Could you check a few things on this model? Use its own coordinates, in mm. A direction names the side the tool comes from. Round coordinates to 2 decimals unless told otherwise and drop trailing zeros. Loops run counter-clockwise (first coordinate to the right, second up) from the corner with the lowest first, then second, coordinate; pieces in that order, holes last.
from build123d import *

# Parameters (mm, degrees)
SKETCH1_W               = 35.2
SKETCH1_H               = 35.2
BOSS_EXTRUDE1_DEPTH     = 34.8
SKETCH2_R               = 11.5
BOSS_EXTRUDE2_DEPTH     = 2
SKETCH3_R               = 2.5
BOSS_EXTRUDE3_DEPTH     = 23
SKETCH4_R               = 1.5
CUT_EXTRUDE1_DEPTH      = 8
MIRROR2_COPY_1_SKETCH_R = 1.5
MIRROR2_COPY_1_DEPTH    = 8
CUT_EXTRUDE2_DEPTH      = 6.96
MIRROR4_COPY_1_DEPTH    = 6.96
CUT_EXTRUDE3_DEPTH      = 6.96
MIRROR6_COPY_1_DEPTH    = 6.96
SKETCH7_R               = 2.5
CUT_EXTRUDE4_DEPTH      = 5
CUT_EXTRUDE6_DEPTH      = 20.88
CUT_EXTRUDE7_DEPTH      = 20.88
CUT_EXTRUDE8_DEPTH      = 20.88
CUT_EXTRUDE9_DEPTH      = 20.88


with BuildPart() as part:
    # Sketch1 → Boss-Extrude1 (new body)
    with BuildSketch(Plane(origin=(0, 0, 0), x_dir=(1, 0, 0), z_dir=(0, 1, 0))):
        Rectangle(SKETCH1_W, SKETCH1_H)
    extrude(amount=BOSS_EXTRUDE1_DEPTH)

    # Sketch2 → Boss-Extrude2 (add)
    with BuildSketch(Plane(origin=(0, 34.8, 0), x_dir=(1, 0, 0), z_dir=(0, 1, 0))):
        Circle(SKETCH2_R)
    extrude(amount=BOSS_EXTRUDE2_DEPTH)

    # Sketch3 → Boss-Extrude3 (add)
    with BuildSketch(Plane(origin=(0, 36.8, 0), x_dir=(1, 0, 0), z_dir=(0, 1, 0))):
        Circle(SKETCH3_R)
    extrude(amount=BOSS_EXTRUDE3_DEPTH)

    # Sketch4 → Cut-Extrude1 (cut)
    with BuildSketch(Plane(origin=(0, 34.8, 0), x_dir=(1, 0, 0), z_dir=(0, 1, 0))):
        with Locations((-13.1, 13.1)):
            Circle(SKETCH4_R)
    cut_extrude1 = extrude(amount=-CUT_EXTRUDE1_DEPTH, mode=Mode.SUBTRACT)

    # Mirror1: Cut-Extrude1 across plane
    add(cut_extrude1.mirror(Plane(origin=(0, 0, 0), x_dir=(0, 0, 1), z_dir=(1, 0, 0))), mode=Mode.SUBTRACT)

    # Mirror2: Cut-Extrude1 across plane
    add(cut_extrude1.mirror(Plane.XY), mode=Mode.SUBTRACT)

    # Mirror2 copy 1 sketch → Mirror2 copy 1 (cut)
    with BuildSketch(Plane(origin=(0, 34.8, 0), x_dir=(-1, 0, 0), z_dir=(0, 1, 0))):
        with Locations((-13.1, 13.1)):
            Circle(MIRROR2_COPY_1_SKETCH_R)
    extrude(amount=-MIRROR2_COPY_1_DEPTH, mode=Mode.SUBTRACT)

    # Sketch5 → Cut-Extrude2 (cut)
    with BuildSketch(Plane(origin=(0, 34.8, 0), x_dir=(1, 0, 0), z_dir=(0, 1, 0))):
        Polygon((-17.6, 17.6), (-14.6, 17.6), (-17.6, 14.6), align=None)
    cut_extrude2 = extrude(amount=-CUT_EXTRUDE2_DEPTH, mode=Mode.SUBTRACT)

    # Mirror3: Cut-Extrude2 across plane
    add(cut_extrude2.mirror(Plane(origin=(0, 0, 0), x_dir=(0, 0, 1), z_dir=(1, 0, 0))), mode=Mode.SUBTRACT)

    # Mirror4: Cut-Extrude2 across plane
    add(cut_extrude2.mirror(Plane.XY), mode=Mode.SUBTRACT)

    # Mirror4 copy 1 sketch → Mirror4 copy 1 (cut)
    with BuildSketch(Plane(origin=(0, 34.8, 0), x_dir=(-1, 0, 0), z_dir=(0, 1, 0))):
        Polygon((-17.6, 17.6), (-14.6, 17.6), (-17.6, 14.6), align=None)
    extrude(amount=-MIRROR4_COPY_1_DEPTH, mode=Mode.SUBTRACT)

    # Sketch6 → Cut-Extrude3 (cut)
    with BuildSketch(Plane.XZ):
        Polygon((-17.6, 17.6), (-14.6, 17.6), (-17.6, 14.6), align=None)
    cut_extrude3 = extrude(amount=-CUT_EXTRUDE3_DEPTH, mode=Mode.SUBTRACT)

    # Mirror5: Cut-Extrude3 across plane
    add(cut_extrude3.mirror(Plane(origin=(0, 0, 0), x_dir=(0, 0, 1), z_dir=(1, 0, 0))), mode=Mode.SUBTRACT)

    # Mirror6: Cut-Extrude3 across plane
    add(cut_extrude3.mirror(Plane.XY), mode=Mode.SUBTRACT)

    # Mirror6 copy 1 sketch → Mirror6 copy 1 (cut)
    with BuildSketch(Plane(origin=(0, 0, 0), x_dir=(-1, 0, 0), z_dir=(0, -1, 0))):
        Polygon((-17.6, 17.6), (-14.6, 17.6), (-17.6, 14.6), align=None)
    extrude(amount=-MIRROR6_COPY_1_DEPTH, mode=Mode.SUBTRACT)

    # Sketch7 → Cut-Extrude4 (cut)
    with BuildSketch(Plane.XZ):
        Circle(SKETCH7_R)
    extrude(amount=-CUT_EXTRUDE4_DEPTH, mode=Mode.SUBTRACT)

    # Sketch8 → Cut-Extrude6 (cut)
    with BuildSketch(Plane(origin=(0, 27.84, 0), x_dir=(1, 0, 0), z_dir=(0, 1, 0))):
        Polygon((-17.6, 17.6), (-13.1, 17.6), (-17.6, 13.1), align=None)
    extrude(amount=-CUT_EXTRUDE6_DEPTH, mode=Mode.SUBTRACT)

    # Sketch9 → Cut-Extrude7 (cut)
    with BuildSketch(Plane(origin=(0, 27.84, 0), x_dir=(1, 0, 0), z_dir=(0, 1, 0))):
        Polygon((17.6, 17.6), (13.1, 17.6), (17.6, 13.1), align=None)
    extrude(amount=-CUT_EXTRUDE7_DEPTH, mode=Mode.SUBTRACT)

    # Sketch10 → Cut-Extrude8 (cut)
    with BuildSketch(Plane(origin=(0, 27.84, 0), x_dir=(1, 0, 0), z_dir=(0, 1, 0))):
        Polygon((17.6, -17.6), (17.6, -13.1), (13.1, -17.6), align=None)
    extrude(amount=-CUT_EXTRUDE8_DEPTH, mode=Mode.SUBTRACT)

    # Sketch11 → Cut-Extrude9 (cut)
    with BuildSketch(Plane(origin=(0, 27.84, 0), x_dir=(1, 0, 0), z_dir=(0, 1, 0))):
        Polygon((-17.6, -17.6), (-17.6, -13.1), (-13.1, -17.6), align=None)
    extrude(amount=-CUT_EXTRUDE9_DEPTH, mode=Mode.SUBTRACT)


solid = part.part
Item 1: We'd pull the mould along Z, two halves only. Please class faces 1 (the cylindrical face through (14.21, 30.86, 14.11)), 2 (the flat face through (-16.1, 31.4, 16.1)), 3 (the flat face through (17.6, 17, 0)): released by +Z, released by -Z, zero draft, split by the parting line, or undercut.
Results list:
face 1: undercut
face 2: released by +Z
face 3: zero draft
Item 2: For faces 4 (the cylindrical face through (-14.21, 30.86, -14.11)), 5 (the flat face through (15.7, 27.84, 15.7)), 6 (the flat face through (-15.7, 27.84, -15.5)), 7 (the flat face through (15.3, 17.5, -15.4)), which set-ups out of +Z, -Z, +X, -X, +Y, -Y let a thin tool reach every point of the face, with its end or its side?
Results list:
face 4: +Y
face 5: +Z, +X
face 6: -Z, -X
face 7: -Z, +X
Item 3: If I drill on line 1 along Z through (x, y) = (-13.1, 31.75); line 2 along Z through (x, y) = (0, 1.85), over which ranges is the centre line in solid material (lowest first)?
Results list:
line 1: z = -17.6 to -14.6, -11.6 to 11.6, 14.6 to 17.6
line 2: z = -17.6 to -2.5, 2.5 to 17.6
Item 4: If we section it at D-D, the plane z = 10: Please give me the cut outline in (x, y).
Results list:
outline: (-17.6, 0) - (17.6, 0) - (17.6, 34.8) - (5.68, 34.8) - (5.68, 36.8) - (-5.68, 36.8) - (-5.68, 34.8) - (-17.6, 34.8) - close
Item 5: If we section it at A-A, the plane x = 0: Please give me the cut outline in (y, z), then the cut area to 3 significant figures.
Results list:
outline: (0, -17.6) - (34.8, -17.6) - (34.8, -11.5) - (36.8, -11.5) - (36.8, -2.5) - (59.8, -2.5) - (59.8, 2.5) - (36.8, 2.5) - (36.8, 11.5) - (34.8, 11.5) - (34.8, 17.6) - (0, 17.6) - (0, 2.5) - (5, 2.5) - (5, -2.5) - (0, -2.5) - close
area: 1,360 mm2
Item 6: If we section it at C-C, the plane y = 10.5: Please give me the cut outline in (x, z).
Results list:
outline: (-17.6, -13.1) - (-13.1, -17.6) - (13.1, -17.6) - (17.6, -13.1) - (17.6, 13.1) - (13.1, 17.6) - (-13.1, 17.6) - (-17.6, 13.1) - close
Item 7: If we section it at B-B, the plane y = 29.5: Please give me the cut outline in (x, z), then the cut area to 3 significant figures.
Results list:
outline: (-17.6, -14.6) - (-14.6, -17.6) - (14.6, -17.6) - (17.6, -14.6) - (17.6, 14.6) - (14.6, 17.6) - (-14.6, 17.6) - (-17.6, 14.6) - close; hole circle Ø3 at (-13.1, -13.1); hole circle Ø3 at (-13.1, 13.1); hole circle Ø3 at (13.1, -13.1); hole circle Ø3 at (13.1, 13.1)
area: 1,190 mm2
Item 8: Will these pins go through, and if not, where does the flat tip stop? pin 1 (4 mm diameter, centred on x = 0, z = 0, fed in from -Y); pin 2 (2 mm diameter, centred on x = 6.5, z = 2.5, fed in from +Y); pin 3 (8 mm diameter, centred on x = -0.5, z = -11.5, fed in from -Y); pin 4 (5 mm diameter, centred on x = -15.5, z = -16, fed in from +Y).
Results list:
pin 1: stops at y = 5
pin 2: stops at y = 36.8
pin 3: stops at y = 0
pin 4: stops at y = 34.8
